from build123d import *

# Parameters (mm, degrees)
F0_W     = 120
F0_H     = 20
F1_DEPTH = 1200
F2_DEPTH = 15
F3_DEPTH = 15
F4_W     = 115
F4_H     = 20
F5_DEPTH = 25
F6_DEPTH = 25
F7_W     = 1000
F7_H     = 20
F8_DEPTH = 10


with BuildPart() as f1:
    # F0 (on Front) → F1 (new body)
    with BuildSketch(Plane.XZ):
        with Locations((60, 10)):
            Rectangle(F0_W, F0_H)
    extrude(amount=F1_DEPTH)

    # F2 (add): a face of the model
    f2_faces = [f1.faces().sort_by_distance(p)[0] for p in [
        (60, -1200, 10),
    ]]
    extrude(f2_faces, amount=F2_DEPTH)

    # F3 (add): a face of the model
    f3_faces = [f1.faces().sort_by_distance(p)[0] for p in [
        (60, 0, 10),
    ]]
    extrude(f3_faces, amount=F3_DEPTH)

    # F4 (on face) → F5 (join)
    with BuildSketch(Plane(origin=(0, 0, 0), x_dir=(0, -1, 0), z_dir=(-1, 0, 0))):
        with Locations((1157.5, 10)):
            Rectangle(F4_W, F4_H)
    extrude(amount=F5_DEPTH)

    # F4 (on face) → F6 (join)
    with BuildSketch(Plane(origin=(0, 0, 0), x_dir=(0, -1, 0), z_dir=(-1, 0, 0))):
        with Locations((42.5, 10)):
            Rectangle(F4_W, F4_H)
    extrude(amount=F6_DEPTH)

    # F7 (on face) → F8 (cut)
    with BuildSketch(Plane(origin=(0, 0, 0), x_dir=(0, -1, 0), z_dir=(-1, 0, 0))):
        with Locations((600, 10)):
            Rectangle(F7_W, F7_H)
    extrude(amount=-F8_DEPTH, mode=Mode.SUBTRACT)


solid = f1.part
Geometry: final body of the model. Coordinates: model frame, mm. A direction names the side the tool comes from. Coordinates: 2 decimals unless noted, no trailing zeros. Order: outer loops, then holes, each group sorted by start corner. A loop starts at its lowest first (then second) coordinate and runs counter-clockwise, first axis right, second up. Notation, with made-up numbers: M -9,-27.75 L 37,-27.75 A23 ccw 37,-0.75 Z; hole C -37.75,-34 d11. An arc over 180 degrees is marked long. One line per question, with ' | ' between items. Start each with the question number.
Item 1: Pin query (flat end, axial travel): pin 1 Ø6 at (y, z) = (-887.5, 16.5) entering from -X; pin 2 Ø5 at (x, y) = (68, -851) entering from -Z. Return the tip coordinate at first contact, or that it passes through.
Item 2: Cut plane B-B, the plane z = 15. Return the cut outline in (x, y).
Item 3: Ray query, probe 1 along Y at (x, z) = (-7, 17); probe 2 along X at (y, z) = (-394, 9.75). Return the intervals inside material, ascending. Write a range as [from, to].
Item 4: Draft query along Y for faces 1 (the flat face through (-25, -42, 10)), 2 (the flat face through (49, -1215, 10)), 3 (the flat face through (49, 15, 10)), 4 (the flat face through (10, -593, 10)). Return one class per face: released by +Y, released by -Y, zero draft, split by the parting line, or undercut.
Item 5: Set-up query: faces 5 (the flat face through (-7, -100, 10)), 6 (the flat face through (65, -591, 20)). Return all of +Z, -Z, +X, -X, +Y, -Y with unobstructed straight access to the full face (end or side cutting, diameter ignored); none if empty.
Item 6: Cut plane A-A, the plane x = -3. Return the cut outline in (y, z).
Item 7: Cut plane C-C, the plane y = -437. Return the cut outline in (x, z), then the cut area to 3 significant figures.
A:
1) pin 1: stops at x = 10 | pin 2: stops at z = 0
2) outline: M -25,-1215 L 120,-1215 L 120,15 L -25,15 L -25,-100 L 10,-100 L 10,-1100 L -25,-1100 Z
3) probe 1: y = [-1215, -1100], [-100, 15] | probe 2: x = [10, 120]
4) face 1: zero draft | face 2: released by -Y | face 3: released by +Y | face 4: undercut
5) face 5: +Z, -Z, -X | face 6: +Z, +X, -X, +Y, -Y
6) outline: M -1215,0 L -1100,0 L -1100,20 L -1215,20 Z; M -100,0 L 15,0 L 15,20 L -100,20 Z
7) outline: M 10,0 L 120,0 L 120,20 L 10,20 Z | area: 2,200 mm2
